Autodesk Inventor part; units mm, degrees
ref_plane "XZ Plane" through (0, 0, 0) normal (0, 1, 0) x (-1, 0, 0)
ref_plane "XY Plane" through (0, 0, 0) normal (0, 0, 1) x (1, 0, 0)
sketch "Sketch1" plane through (0, 0, 0) normal (0, 1, 0) x (-1, 0, 0)
  circle A0 centre (0, 0) radius 39.37
  dimension "d0" = 78.74
extrude "Extrusion1" add sketch "Sketch1" along normal blind 127
sketch "Sketch2" plane through (0, 127, 0) normal (0, 1, 0) x (1, 0, 0)
  circle A0 centre (0, 0) radius 38.1
  dimension "d3" = 76.2
extrude "Extrusion2" cut sketch "Sketch2" against normal blind 127
sketch "Sketch3" plane through (0, 0, 0) normal (0, -1, 0) x (1, 0, 0)
  circle A0 centre (0, 0) radius 39.37
extrude "Extrusion3" add sketch "Sketch3" along normal blind 33.02
sketch "Sketch4" plane through (0, 0, 0) normal (1, 0, 0) x (0, 1, 0)
  line L0 (-33.02, 39.37) -> (-33.02, -39.37)
  line L1 (0, 39.2884) -> (-33.02, 39.2884)
  line L2 (-33.02, 39.2884) -> (-33.02, -39.37)
  line L3 (-33.02, -39.37) -> (0, -39.37)
  line L4 (0, -39.37) -> (0, 39.2884)
  point P0 (0, 0)
extrude "Extrusion4" add sketch "Sketch4" against normal blind 67.31
ref_plane "Work Plane1" through (39.37, 0, 0) normal (1, 0, 0) x (0, 1, 0)
sketch "Sketch5" plane through (39.37, 0, 0) normal (1, 0, 0) x (0, 1, 0)
  line L0 (-3.1755, 0) -> (-31.1155, 0)
  line L1 (-31.1155, 0) -> (-31.1155, 29.21)
  line L2 (-31.1155, 29.21) -> (-3.1755, 29.21)
  line L3 (-3.1755, 29.21) -> (-3.1755, 0)
  line L4 (-3.1755, 0) -> (-31.1155, 0)
  line L5 (-31.1155, 0) -> (-31.1155, -29.845)
  line L6 (-31.1155, -29.845) -> (-3.1755, -29.845)
  line L7 (-3.1755, -29.845) -> (-3.1755, 0)
  point P0 (0, 0)
  dimension "d10" = 27.94
  dimension "d11" = 29.21
  dimension "d12" = 27.94
  dimension "d13" = 29.845
extrude "Extrusion5" cut sketch "Sketch5" against normal blind 103.8225
sketch "Sketch6" plane through (0, 0, 0) normal (0, 0, 1) x (1, 0, 0)
  line L0 (39.37, -33.02) -> (39.37, 127)
  line L1 (39.37, -2.744) -> (13.0341, -2.744)
  line L2 (13.0341, -2.744) -> (-104.9586, 63.1124)
  line L3 (13.0341, -6.86) -> (-27.6059, -6.86)
  line L4 (-27.6059, -6.86) -> (-27.6059, -24.64)
  line L5 (-27.6059, -24.64) -> (13.0341, -24.64)
  line L6 (13.0341, -24.64) -> (13.0341, -6.86)
  point P0 (0, 0)
  dimension "d16" = 40.64
  dimension "d17" = 17.78
extrude "Extrusion6" cut sketch "Sketch6" along normal blind 102.5525
sketch "Sketch7" plane through (0, 0, 0) normal (0, 0, 1) x (1, 0, 0)
  point P0 (0, 0)
sketch "Sketch8" plane through (0, 0, 0) normal (0, 0, 1) x (1, 0, 0)
  point P0 (0, 0)
sketch "Sketch9" plane through (0, 0, 0) normal (0, 0, 1) x (1, 0, 0)
  point P0 (0, 0)
sketch "Sketch10" plane through (0, 0, 0) normal (0, 0, 1) x (1, 0, 0)
  line L0 (0, 7.3743) -> (-17.78, 7.3743)
  line L1 (-17.78, 7.3743) -> (-17.78, 30.2343)
  line L2 (-17.78, 30.2343) -> (0, 30.2343)
  line L3 (0, 30.2343) -> (0, 7.3743)
  point P0 (0, 0)
  dimension "d20" = 17.78
  dimension "d21" = 22.86
extrude "Extrusion7" cut sketch "Sketch10" against normal blind 102.5525
sketch "Sketch11" plane through (0, 0, 0) normal (1, 0, 0) x (0, 1, 0)
  line L0 (127, -39.37) -> (127, 39.37)
  line L1 (127, 0) -> (68.58, 0)
  line L2 (68.58, 0) -> (68.58, 25.4)
  line L3 (59.5338, 0) -> (59.5338, -25.4)
  line L4 (59.5338, -25.4) -> (54.4538, -25.4)
  line L5 (54.4538, -25.4) -> (54.4538, -27.94)
  line L6 (54.4538, -27.94) -> (59.5338, -27.94)
  line L7 (59.5338, -27.94) -> (59.5338, -25.4)
  line L8 (59.5338, 25.4) -> (54.4538, 25.4)
  line L9 (54.4538, 25.4) -> (54.4538, 27.94)
  line L10 (54.4538, 27.94) -> (59.5338, 27.94)
  line L11 (59.5338, 27.94) -> (59.5338, 25.4)
  line L12 (15.2971, -27.94) -> (10.2171, -27.94)
  line L13 (10.2171, -27.94) -> (10.2171, -25.4)
  line L14 (10.2171, -25.4) -> (15.2971, -25.4)
  line L15 (15.2971, -25.4) -> (15.2971, -27.94)
  line L16 (15.2971, 25.4) -> (10.2171, 25.4)
  line L17 (10.2171, 25.4) -> (10.2171, 27.94)
  line L18 (10.2171, 27.94) -> (15.2971, 27.94)
  line L19 (15.2971, 27.94) -> (15.2971, 25.4)
  point P0 (0, 0)
  dimension "d24" = 58.42
  dimension "d25" = 25.4
  dimension "d26" = 25.4
  dimension "d27" = 5.08
  dimension "d28" = 2.54
  dimension "d29" = 5.08
  dimension "d30" = 2.54
  dimension "d31" = 5.08
  dimension "d32" = 2.54
extrude "Extrusion8" cut sketch "Sketch11" against normal blind 83.185
sketch "Sketch12" plane through (0, -33.02, 0) normal (0, -1, 0) x (1, 0, 0)
  point P0 (0, 0)
sketch "Sketch13" plane through (0, -33.02, 0) normal (0, -1, 0) x (1, 0, 0)
  circle A0 centre (0, 0) radius 39.37
  dimension "d35" = 78.74
extrude "Extrusion9" add sketch "Sketch13" along normal blind 5.08
sketch "Sketch14" plane through (0, -33.02, 0) normal (0, -1, 0) x (1, 0, 0)
  circle A0 centre (0, 0) radius 39.37
  line L0 (0, -39.37) -> (-67.31, -39.37)
  line L1 (0, 39.37) -> (-67.31, 39.37)
  line L2 (-67.31, 39.37) -> (-67.31, -39.37)
  line L3 (-67.31, -39.37) -> (0, -39.37)
  line L4 (0, -39.37) -> (0, 39.37)
extrude "Extrusion10" add sketch "Sketch14" along normal blind 5.08 contours A0 L0 L2 L1
sketch "Sketch15" plane through (39.37, 0, 0) normal (1, 0, 0) x (0, 1, 0)
  line L0 (-31.1155, 29.21) -> (-31.1155, -29.845)
  line L1 (-31.1155, 29.21) -> (-36.1955, 29.21)
  line L2 (-36.1955, 29.21) -> (-36.1955, -29.845)
  line L3 (-36.1955, -29.845) -> (-31.1155, -29.845)
  line L4 (-31.1155, -29.845) -> (-31.1155, 29.21)
  point P0 (0, 0)
  dimension "d40" = 5.08
  dimension "d41" = 59.055
extrude "Extrusion11" cut sketch "Sketch15" against normal blind 104.14
properties part number "_3DPrint"
Source: CAD feature listing. Evaluate the final solid. Frame: model axes, mm. A direction names the side the tool comes from. Round coordinates to 2 decimals unless told otherwise and drop trailing zeros. Loops run counter-clockwise (first coordinate to the right, second up) from the corner with the lowest first, then second, coordinate; pieces in that order, holes last. Notation, with made-up numbers: M -15,-12 L 42,-12 A13 ccw 42,4 Z; hole C 88.25,-36.5 d6. An arc over 180 degrees is marked long. Use a Markdown table: item, result. Add a question column.
1. Section query C-C on z = 0. Return the cut outline in (x, y), then the cut area to 3 significant figures.
2. Mould query, pull axis Y, two halves, no side actions, for faces 1 (the flat face through (-7, -6.86, 34)), 2 (the flat face through (-64.452, -17, 0)), 3 (the flat face through (-42, -16, 39.288)), 4 (the flat face through (-15, -38.1, 1)). Classes: pulls with the +Y half, pulls with the -Y half, needs draft (parallel to the pull), parting line crosses it, or undercut.
3. Section query A-A on y = 57.5. Return the cut outline in (x, z), then the cut area to 3 significant figures.
4. Reachability of faces 5 (the flat face through (-29, -19, 29.21)), 6 (the cylindrical face through (18.167, 63.95, 34.928)), 7 (the flat face through (-8, -24.64, 34)) from +Z, -Z, +X, -X, +Y, -Y: full face, straight path, thin tool, end or side. Return the list, or none.
5. Line query: line 1 (Z direction, x = -61, y = -9.5) (3 decimals); line 2 (Z direction, x = 0, y = 74); line 3 (Y direction, x = -55.5, z = -10.5). Output: solid intervals per line, ascending.
6. Section query D-D on z = 32.5. Return the cut outline in (x, y), then the cut area to 3 significant figures.
7. Contact query for flat-ended pins moving along their axis: P1, Ø1.5, axis at x = -26.5, y = 13.5, coming from the +Z side; P2, Ø1.5, axis at y = -34.5, z = -8.5, coming from the +X side; P3, Ø0.6, axis at x = -26.5, y = 12, coming from the -Z side; P4, Ø2, axis at x = 27.5, z = 30.5, coming from the -Y side. Output: stop coordinate, or through.
Reported:
| question | item | result |
|---|---|---|
| 1 | outline | M -67.31,-38.1 L 39.37,-38.1 L 39.37,-36.2 L -64.77,-36.2 L -64.77,-31.12 L -64.45,-31.12 L -64.45,-3.18 L 39.37,-3.18 L 39.37,127 L 38.1,127 L 38.1,0 L -38.1,0 L -38.1,127 L -39.37,127 L -39.37,0 L -67.31,0 Z |
| 1 | area | 957 mm² |
| 2 | face 1 | undercut |
| 2 | face 2 | undercut |
| 2 | face 3 | needs draft |
| 2 | face 4 | pulls with the -Y half |
| 3 | outline | M -30.08,-25.4 L -28.4,-25.4 A38.1 cw -28.4,25.4 L -30.08,25.4 A39.37 ccw Z; M -27.74,-27.94 A39.37 ccw long -27.74,27.94 L -25.9,27.94 A38.1 cw long -25.9,-27.94 Z |
| 3 | area | 300 mm² |
| 4 | face 5 | +X |
| 4 | face 6 | +Y |
| 4 | face 7 | +Z |
| 5 | line 1 | z = -39.37 to -29.845, 29.21 to 39.288 |
| 5 | line 2 | z = -39.37 to -38.1, 38.1 to 39.37 |
| 5 | line 3 | y = -38.1 to -36.2, -3.18 to 0 |
| 6 | outline | M -67.31,-38.1 L 22.22,-38.1 L 22.22,127 L 19.88,127 L 19.88,0 L -19.88,0 L -19.88,127 L -22.22,127 L -22.22,0 L -67.31,0 Z; hole M -27.61,-24.64 L 13.03,-24.64 L 13.03,-6.86 L -27.61,-6.86 Z |
| 6 | area | 3,280 mm² |
| 7 | P1 | stops at z = 29.78 |
| 7 | P2 | stops at x = -64.77 |
| 7 | P3 | stops at z = -29.39 |
| 7 | P4 | passes through |
